from build123d import *

# Parameters (mm, degrees)
CROQUIS2_W                 = 25
CROQUIS2_H                 = 15
SALIENTE_EXTRUIR1_DEPTH    = 40
CROQUIS3_W                 = 15
CROQUIS3_H                 = 15
CORTAR_EXTRUIR1_DEPTH      = 20
REDONDEO1_R                = 1
REDONDEO2_R                = 1
CORTAR_EXTRUIR2_DEPTH      = 18
CORTAR_EXTRUIR2_DEPTH_BACK = 3
CROQUIS4_R                 = 3.15
CROQUIS6_W                 = 5
CROQUIS6_H                 = 3
SALIENTE_EXTRUIR2_DEPTH    = 5
REDONDEO3_R                = 2
CROQUIS8_R                 = 1.5
CORTAR_EXTRUIR3_DEPTH      = 15
CROQUIS9_W                 = 5
CROQUIS9_H                 = 3
SALIENTE_EXTRUIR3_DEPTH    = 5
CORTAR_EXTRUIR4_REACH      = 43.611
CROQUIS10_R                = 1.5
REDONDEO4_R                = 2
REDONDEO5_R                = 0.5
REDONDEO6_R                = 0.5


with BuildPart() as part:
    # Croquis2 → Saliente-Extruir1 (new body)
    with BuildSketch(Plane(origin=(0, 0, 0), x_dir=(1, 0, 0), z_dir=(0, 1, 0))):
        Rectangle(CROQUIS2_W, CROQUIS2_H)
    extrude(amount=SALIENTE_EXTRUIR1_DEPTH)

    # Croquis3 → Cortar-Extruir1 (cut)
    with BuildSketch(Plane(origin=(0, 40, 0), x_dir=(1, 0, 0), z_dir=(0, 1, 0))):
        Rectangle(CROQUIS3_W, CROQUIS3_H)
    extrude(amount=-CORTAR_EXTRUIR1_DEPTH, mode=Mode.SUBTRACT)

    # Redondeo1
    redondeo1_edges = [part.edges().sort_by_distance(p)[0] for p in [
        (7.5, 20, 0),
        (-7.5, 20, 0),
    ]]
    fillet(redondeo1_edges, radius=REDONDEO1_R)

    # Redondeo2
    redondeo2_edges = [part.edges().sort_by_distance(p)[0] for p in [
        (7.5, 40, 0),
        (-7.5, 40, 0),
    ]]
    fillet(redondeo2_edges, radius=REDONDEO2_R)

    # Croquis4 → Cortar-Extruir2 (cut, two sides: drawn at the far end of the back side and taken through both)
    with BuildSketch(Plane(origin=(-7.5, 0, 0), x_dir=(0, 0, -1), z_dir=(1, 0, 0)).offset(-CORTAR_EXTRUIR2_DEPTH_BACK)):
        with Locations(Location((0, 35.5, 0), (0, 0, 180))):
            Circle(CROQUIS4_R)
    extrude(amount=CORTAR_EXTRUIR2_DEPTH + CORTAR_EXTRUIR2_DEPTH_BACK, mode=Mode.SUBTRACT)

    # Croquis6 → Saliente-Extruir2 (add)
    with BuildSketch(Plane(origin=(12.5, 0, 0), x_dir=(0, 0, -1), z_dir=(1, 0, 0))):
        with Locations((0, 1.5)):
            Rectangle(CROQUIS6_W, CROQUIS6_H)
    extrude(amount=SALIENTE_EXTRUIR2_DEPTH)

    # Redondeo3
    redondeo3_edges = [part.edges().sort_by_distance(p)[0] for p in [
        (17.5, 1.5, -2.5),
        (17.5, 1.5, 2.5),
    ]]
    fillet(redondeo3_edges, radius=REDONDEO3_R)

    # Croquis8 → Cortar-Extruir3 (cut)
    with BuildSketch(Plane(origin=(0, 3, 0), x_dir=(1, 0, 0), z_dir=(0, 1, 0))):
        with Locations(Location((15, 0, 0), (0, 0, 270))):
            Circle(CROQUIS8_R)
    extrude(amount=-CORTAR_EXTRUIR3_DEPTH, mode=Mode.SUBTRACT)

    # Croquis9 → Saliente-Extruir3 (add)
    with BuildSketch(Plane.ZY.offset(12.5)):
        with Locations((0, 1.5)):
            Rectangle(CROQUIS9_W, CROQUIS9_H)
    extrude(amount=SALIENTE_EXTRUIR3_DEPTH)

    # Croquis10 → Cortar-Extruir4 (cut, up to next)
    with BuildSketch(Plane(origin=(0, 3, 0), x_dir=(1, 0, 0), z_dir=(0, 1, 0)), mode=Mode.PRIVATE) as cortar_extruir4_sk1:
        with Locations(Location((-15, 0, 0), (0, 0, 270))):
            Circle(CROQUIS10_R)
    cortar_extruir4_tool1 = extrude(cortar_extruir4_sk1.sketch, amount=-CORTAR_EXTRUIR4_REACH, mode=Mode.PRIVATE) & part.part
    add(cortar_extruir4_tool1.solids().sort_by_distance((-15, 3, 0))[0], mode=Mode.SUBTRACT)

    # Redondeo4
    redondeo4_edges = [part.edges().sort_by_distance(p)[0] for p in [
        (-17.5, 1.5, 2.5),
        (-17.5, 1.5, -2.5),
    ]]
    fillet(redondeo4_edges, radius=REDONDEO4_R)

    # Redondeo5
    redondeo5_edges = [part.edges().sort_by_distance(p)[0] for p in [
        (12.5, 1.5, -2.5),
        (12.5, 3, 0),
        (12.5, 1.5, 2.5),
        (-12.5, 1.5, 2.5),
        (-12.5, 3, 0),
        (-12.5, 1.5, -2.5),
    ]]
    fillet(redondeo5_edges, radius=REDONDEO5_R)

    # Redondeo6
    redondeo6_edges = [part.edges().sort_by_distance(p)[0] for p in [
        (-12.5, 40, 0),
        (-10.5, 40, 7.5),
        (0, 20, -7.5),
        (0, 20, 7.5),
        (7.5, 30, -7.5),
        (7.5, 30, 7.5),
        (-7.5, 30, 7.5),
        (-7.5, 30, -7.5),
        (7.207106781, 20.292893219, -7.5),
        (7.207106781, 20.292893219, 7.5),
        (-7.207106781, 20.292893219, 7.5),
        (-7.207106781, 20.292893219, -7.5),
        (10.5, 40, 7.5),
        (7.792893219, 39.707106781, 7.5),
        (-7.792893219, 39.707106781, 7.5),
        (-10.5, 40, -7.5),
        (7.792893219, 39.707106781, -7.5),
        (-7.792893219, 39.707106781, -7.5),
        (12.5, 40, 0),
        (10.5, 40, -7.5),
    ]]
    fillet(redondeo6_edges, radius=REDONDEO6_R)


solid = part.part
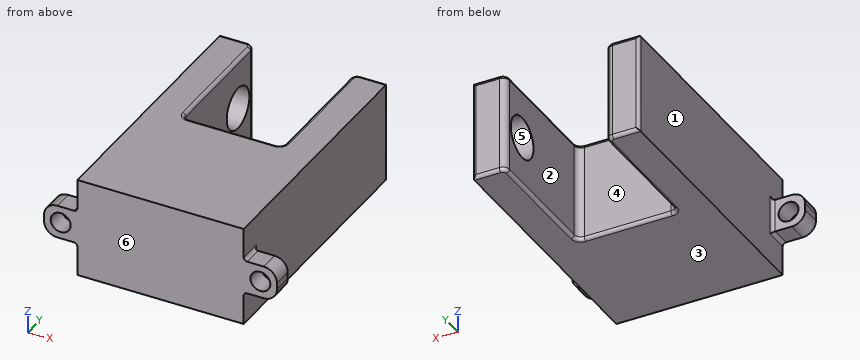
CAD build for the part. Positions are in the model's coordinates, mm. Face numbers are marked on the shaded views. A direction names the side the tool comes from. Round coordinates to 2 decimals unless told otherwise and drop trailing zeros. Loops run counter-clockwise (first coordinate to the right, second up) from the corner with the lowest first, then second, coordinate; pieces in that order, holes last.
(1) Which spindle directions (+Z, -Z, +X, -X, +Y, -Y) get a long thin tool onto all of the face, cutting with end or side? Do the marked faces 4, 5 and 6. Say none if no direction does.
(2) Cut at B-B (y = 2). Give the cut face in (x, z), plus the area to 3 significant figures.
(3) Cut at D-D (x = -9). Give the cut face in (y, z), plus the area to 3 significant figures.
(4) Two-plate mould, pull along X, no slides. Class the marked faces 1, 2 and 3: +X half, -X half, draft (parallel to the pull), parting line (faces both ways), or undercut.
(5) Drop flat-ended pins along their axis: pin 1 (4.5 mm diameter, centred on y = 17.5, z = 2.5, fed in from -X); pin 2 (1.2 mm diameter, centred on x = 15, y = 1, fed in from -Z); pin 3 (8 mm diameter, centred on y = 35.5, z = 0, fed in from +X). Give the stop position or say it passes through.
(6) Cut at C-C (y = 35.5). Give the cut face in (x, z).
(7) Cut at A-A (x = 15). Give the cut face in (y, z), plus the area to 3 significant figures.
(8) Wall check: line 1 along X through (y, z) = (1.05, 0); line 2 along Y through (x, z) = (8.85, 0); line 3 along X through (y, z) = (34, 1.75). Give the ranges that are in metal, low to high.
Findings below:
1. face 4: +Z, -Z, +Y
1. face 5: none
1. face 6: +Z, -Z, +X, -X, -Y
2. outline: (-17.5, -0.5) arc R2 ccw to (-15.5, -2.5) - (-13, -2.5) arc R0.5 cw to (-12.5, -3) - (-12.5, -7.5) - (12.5, -7.5) - (12.5, -3) arc R0.5 cw to (13, -2.5) - (15.5, -2.5) arc R2 ccw to (17.5, -0.5) - (17.5, 0.5) arc R2 ccw to (15.5, 2.5) - (13, 2.5) arc R0.5 cw to (12.5, 3) - (12.5, 7.5) - (-12.5, 7.5) - (-12.5, 3) arc R0.5 cw to (-13, 2.5) - (-15.5, 2.5) arc R2 ccw to (-17.5, 0.5) - close; hole circle Ø3 at (-15, 0); hole circle Ø3 at (15, 0)
2. area: 408 mm2
3. outline: (0, -7.5) - (39.5, -7.5) arc R0.5 ccw to (40, -7) - (40, 7) arc R0.5 ccw to (39.5, 7.5) - (0, 7.5) - close; hole circle Ø6.3 at (35.5, 0)
3. area: 569 mm2
4. face 1: -X half
4. face 2: undercut
4. face 3: draft
5. pin 1: stops at x = -12.5
5. pin 2: stops at z = -2.5
5. pin 3: stops at x = 12.5
6. outline: (-12.5, -7.5) - (-8, -7.5) arc R0.5 ccw to (-7.5, -7) - (-7.5, -3.15) - (-10.5, -3.15) - (-10.5, 3.15) - (-7.5, 3.15) - (-7.5, 7) arc R0.5 ccw to (-8, 7.5) - (-12.5, 7.5) - close; (7.5, -7) arc R0.5 ccw to (8, -7.5) - (12.5, -7.5) - (12.5, 7.5) - (8, 7.5) arc R0.5 ccw to (7.5, 7) - (7.5, 3.15) - (10.5, 3.15) - (10.5, -3.15) - (7.5, -3.15) - close
7. outline: (0, -2.5) - (3, -2.5) - (3, -1.5) - (0, -1.5) - close; (0, 1.5) - (3, 1.5) - (3, 2.5) - (0, 2.5) - close
7. area: 6.00 mm2
8. line 1: x = -17.5 to -16.5, -13.5 to 13.5, 16.5 to 17.5
8. line 2: y = 0 to 32.35, 38.65 to 40
8. line 3: x = -12.5 to -10.5, 10.5 to 12.5
